Here's the drawing with two shaded views (mm, measured from the low corner). I have some questions. A direction names the side the tool comes from. Give positions to 0.01 mm unless a question says otherwise; leave off trailing zeros. Loops run counter-clockwise (first coordinate to the right, second up) from the corner with the lowest first, then second, coordinate; pieces in that order, holes last. Notation, with made-up numbers: M 5,43 L 17,43 A21 cw 17,55 Z; hole C 80.5,82 d5. An arc over 180 degrees is marked long. Use a Markdown table: item, result. Add a question column.
1) Suppose I cut it at C-C on y = 12. List the corners of the cut face in (x, z) for me.
2) Which directions (+Z, -Z, +X, -X, +Y, -Y) give clear straight access to the entire face, cutting with the end or side of a thin tool? Please do the marked faces 4 and 5.
3) Will these pins go through, and if not, where does the flat tip stop? pin 1 Ø1.5 at (x, y) = (9.975, 16.975) entering from +Z; pin 2 Ø1.5 at (x, z) = (14.5, 3.5) entering from +Y; pin 3 Ø4 at (x, y) = (16.975, 9.975) entering from +Z; pin 4 Ø1.8 at (x, y) = (11, 9.5) entering from +Z.
4) Suppose I cut it at B-B on x = 2.5. List the corners of the cut face in (y, z) for me, and give its area (3 significant figures).
5) Suppose I cut it at D-D on z = 1.25. List the corners of the cut face in (x, y) for me (3 decimals).
6) We'd pull the mould along Y, two halves only. Please class the marked faces 1, 2 and 3: +Y half, -Y half, draft (parallel to the pull), parting line (faces both ways), or undercut.
7) If I drill on line 1 along Y through (x, z) = (10, 1.4); line 2 along X through (y, z) = (9, 1.15); line 3 along Z through (x, y) = (4.5, 12.75), over which ranges is the centre line in solid material (lowest first)? Write a range as [from, to].
8) Suppose I cut it at A-A on x = 10.25. List the corners of the cut face in (y, z) for me, and give its area (3 significant figures).
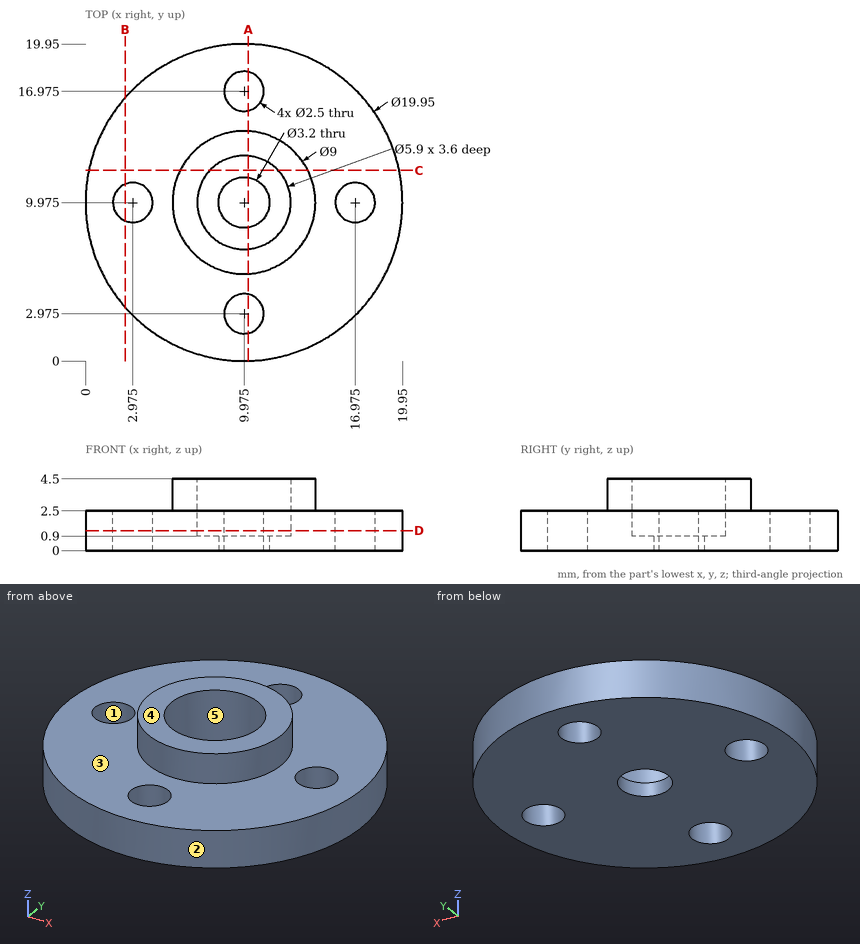
Answer block:
| question | item | result |
|---|---|---|
| 1 | outline | M 0.21,0 L 19.74,0 L 19.74,2.5 L 13.99,2.5 L 13.99,4.5 L 12.12,4.5 L 12.12,0.9 L 7.83,0.9 L 7.83,4.5 L 5.96,4.5 L 5.96,2.5 L 0.21,2.5 Z |
| 2 | face 4 | +Z, +X, -X, +Y, -Y |
| 2 | face 5 | +Z |
| 3 | pin 1 | passes through |
| 3 | pin 2 | stops at y = 12.42 |
| 3 | pin 3 | stops at z = 2.5 |
| 3 | pin 4 | stops at z = 0.9 |
| 4 | outline | M 3.37,0 L 8.82,0 L 8.82,2.5 L 3.37,2.5 Z; M 11.13,0 L 16.58,0 L 16.58,2.5 L 11.13,2.5 Z |
| 4 | area | 27.2 mm^2 |
| 5 | outline | C 9.975,9.975 d19.95; hole C 2.975,9.975 d2.5; hole C 9.975,9.975 d5.9; hole C 9.975,2.975 d2.5; hole C 9.975,16.975 d2.5; hole C 16.975,9.975 d2.5 |
| 6 | face 1 | undercut |
| 6 | face 2 | parting line |
| 6 | face 3 | draft |
| 7 | line 1 | y = [0, 1.73], [4.22, 7.03], [12.92, 15.73], [18.22, 19.95] |
| 7 | line 2 | x = [0.05, 2.19], [3.76, 7.19], [12.76, 16.19], [17.76, 19.9] |
| 7 | line 3 | z = [0, 2.5] |
| 8 | outline | M 0,0 L 1.76,0 L 1.76,2.5 L 0,2.5 Z; M 4.19,0 L 8.4,0 L 8.4,0.9 L 7.04,0.9 L 7.04,4.5 L 5.48,4.5 L 5.48,2.5 L 4.19,2.5 Z; M 11.55,0 L 15.76,0 L 15.76,2.5 L 14.47,2.5 L 14.47,4.5 L 12.91,4.5 L 12.91,0.9 L 11.55,0.9 Z; M 18.19,0 L 19.95,0 L 19.95,2.5 L 18.19,2.5 Z |
| 8 | area | 31.6 mm^2 |
